```python
from build123d import *

# Parameters (mm, degrees)
SKETCH1_R                  = 1.79959
BASE_FLANGE1_DEPTH         = 2.3622
SKETCHED_START             = -88.9
SKETCHED_BEND1_OUTLINE_W   = 12.7
SKETCHED_BEND1_OUTLINE_H   = 2.3622
SKETCHED_BEND1_DEPTH       = 60.4012
SKETCHED_START_2           = -28.197410712
SKETCHED_BEND1_2_OUTLINE_W = 12.7
SKETCHED_BEND1_2_OUTLINE_H = 61.224283884
SKETCHED_BEND1_2_OUTLINE_R = 1.79959
SKETCHED_BEND1_2_DEPTH     = 2.060810712
SKETCHED_START_3           = -28.4988
SKETCHED_BEND1_3_OUTLINE_W = 12.7
SKETCHED_BEND1_3_OUTLINE_H = 61.224283884
SKETCHED_BEND1_3_OUTLINE_R = 1.79959
SKETCHED_BEND1_3_DEPTH     = 3.0988
SKETCHED_START_4           = 38.1
SKETCHED_BEND1_4_DEPTH     = 12.7
CUT_EXTRUDE1_REACH         = 88.233
SKETCH7_R                  = 1.55


with BuildPart() as part:
    # Base-Flange1: sheet metal written as solids
    # Sketch1 → Base-Flange1 (new body)
    with BuildSketch(Plane(origin=(0, 0, 0), x_dir=(1, 0, 0), z_dir=(0, 1, 0))):
        Polygon((50.8, 88.9), (50.8, 0), (0, 0), (0, 25.4), (38.1, 25.4), (38.1, 88.9), align=None)
        with Locations(Location((45.06468, 81.50352, 0), (0, 0, 270))):
            Circle(SKETCH1_R, mode=Mode.SUBTRACT)
        with Locations(Location((44.45, 35.56, 0), (0, 0, 270))):
            Circle(SKETCH1_R, mode=Mode.SUBTRACT)
    extrude(amount=-BASE_FLANGE1_DEPTH)

    # Sketched Bend1: read off the stored shape, not the designer's step
    # Sketched Bend1 outline → Sketched Bend1 (cut)
    with BuildSketch(Plane.XY.offset(SKETCHED_START)):
        with Locations((44.45, -1.1811)):
            Rectangle(SKETCHED_BEND1_OUTLINE_W, SKETCHED_BEND1_OUTLINE_H)
    extrude(amount=SKETCHED_BEND1_DEPTH, mode=Mode.SUBTRACT)

    # Sketched Bend1 2 outline → Sketched Bend1 2 (add)
    with BuildSketch(Plane.XY.offset(SKETCHED_START_2)):
        with Locations((44.45, -32.974341942)):
            Rectangle(SKETCHED_BEND1_2_OUTLINE_W, SKETCHED_BEND1_2_OUTLINE_H)
        with Locations((45.06468, -56.190003884)):
            Circle(SKETCHED_BEND1_2_OUTLINE_R, mode=Mode.SUBTRACT)
        with Locations((44.45, -10.246483884)):
            Circle(SKETCHED_BEND1_2_OUTLINE_R, mode=Mode.SUBTRACT)
    extrude(amount=SKETCHED_BEND1_2_DEPTH)

    # Sketched Bend1 3 outline → Sketched Bend1 3 (add)
    with BuildSketch(Plane.XY.offset(SKETCHED_START_3)):
        with Locations((44.45, -32.974341942)):
            Rectangle(SKETCHED_BEND1_3_OUTLINE_W, SKETCHED_BEND1_3_OUTLINE_H)
        with Locations((45.06468, -56.190003884)):
            Circle(SKETCHED_BEND1_3_OUTLINE_R, mode=Mode.SUBTRACT)
        with Locations((44.45, -10.246483884)):
            Circle(SKETCHED_BEND1_3_OUTLINE_R, mode=Mode.SUBTRACT)
    extrude(amount=SKETCHED_BEND1_3_DEPTH)

    # Sketched Bend1 4 outline → Sketched Bend1 4 (cut)
    with BuildSketch(Plane.YZ.offset(SKETCHED_START_4)):
        with BuildLine():
            ThreePointArc((0, -25.4), (-0.907617506, -27.591182494), (-3.0988, -28.4988))
            Line((-3.0988, -28.4988), (0, -28.4988))
            Line((0, -28.4988), (0, -25.4))
        make_face()
        with BuildLine():
            Line((-63.586483884, -26.1366), (-3.0988, -26.1366))
            ThreePointArc((-3.0988, -26.1366), (-2.577945145, -25.920854855), (-2.3622, -25.4))
            Line((-2.3622, -25.4), (-63.586483884, -25.4))
            Line((-63.586483884, -25.4), (-63.586483884, -26.1366))
        make_face()
    extrude(amount=SKETCHED_BEND1_4_DEPTH, mode=Mode.SUBTRACT)

    # Sketch7 → Cut-Extrude1 (cut, up to next)
    with BuildSketch(Plane(origin=(0, 0, 0), x_dir=(1, 0, 0), z_dir=(0, 1, 0)), mode=Mode.PRIVATE) as cut_extrude1_sk1:
        with Locations(Location((45.78, 20.828, 0), (0, 0, 270))):
            Circle(SKETCH7_R)
    cut_extrude1_tool1 = extrude(cut_extrude1_sk1.sketch, amount=-CUT_EXTRUDE1_REACH, mode=Mode.PRIVATE) & part.part
    # Sketch7 → Cut-Extrude1 (cut, up to next)
    with BuildSketch(Plane(origin=(0, 0, 0), x_dir=(1, 0, 0), z_dir=(0, 1, 0)), mode=Mode.PRIVATE) as cut_extrude1_sk2:
        with Locations(Location((5.08, 4.528, 0), (0, 0, 270))):
            Circle(SKETCH7_R)
    cut_extrude1_tool2 = extrude(cut_extrude1_sk2.sketch, amount=-CUT_EXTRUDE1_REACH, mode=Mode.PRIVATE) & part.part
    # Sketch7 → Cut-Extrude1 (cut, up to next)
    with BuildSketch(Plane(origin=(0, 0, 0), x_dir=(1, 0, 0), z_dir=(0, 1, 0)), mode=Mode.PRIVATE) as cut_extrude1_sk3:
        with Locations(Location((45.78, 4.528, 0), (0, 0, 270))):
            Circle(SKETCH7_R)
    cut_extrude1_tool3 = extrude(cut_extrude1_sk3.sketch, amount=-CUT_EXTRUDE1_REACH, mode=Mode.PRIVATE) & part.part
    # Sketch7 → Cut-Extrude1 (cut, up to next)
    with BuildSketch(Plane(origin=(0, 0, 0), x_dir=(1, 0, 0), z_dir=(0, 1, 0)), mode=Mode.PRIVATE) as cut_extrude1_sk4:
        with Locations(Location((5.08, 20.828, 0), (0, 0, 270))):
            Circle(SKETCH7_R)
    cut_extrude1_tool4 = extrude(cut_extrude1_sk4.sketch, amount=-CUT_EXTRUDE1_REACH, mode=Mode.PRIVATE) & part.part
    add(cut_extrude1_tool1.solids().sort_by_distance((45.78, 0, -20.828))[0], mode=Mode.SUBTRACT)
    add(cut_extrude1_tool2.solids().sort_by_distance((5.08, 0, -4.528))[0], mode=Mode.SUBTRACT)
    add(cut_extrude1_tool3.solids().sort_by_distance((45.78, 0, -4.528))[0], mode=Mode.SUBTRACT)
    add(cut_extrude1_tool4.solids().sort_by_distance((5.08, 0, -20.828))[0], mode=Mode.SUBTRACT)


solid = part.part
```
Verification items for the finished model (mm, model axes). A direction names the side the tool comes from. Coordinates: 2 decimals unless noted, no trailing zeros. Order: outer loops, then holes, each group sorted by start corner. A loop starts at its lowest first (then second) coordinate and runs counter-clockwise, first axis right, second up. Notation, with made-up numbers: (87, -6) - (146, -6) arc R29 ccw to (146, 32) - close; hole circle Ø11 at (2.25, -26). An arc over 180 degrees is marked (long way). Return JSON: item names as keys, results as strings.
(1) Go/stop test with flat-tipped pins: pin 1 (14 mm diameter, centred on x = 46, y = -41.5, fed in from +Z); pin 2 (2 mm diameter, centred on x = 45.06, y = -56.19, fed in from +Z); pin 3 (3.5 mm diameter, centred on x = 5.08, z = -20.828, fed in from -Y); pin 4 (1.9 mm diameter, centred on x = 12.5, y = -1.5, fed in from -Z). Record where each tip stops, or that it passes through.
Filled sheet:
{"pin 1": "stops at z = -26.14", "pin 2": "passes through", "pin 3": "stops at y = -2.36", "pin 4": "stops at z = -25.4"}
(2) Section check B-B, the plane z = -5.25. Record the cut outline in (x, y), and give its area (3 significant figures).
Filled sheet:
{"outline": "(0, -2.36) - (3.71, -2.36) - (3.71, 0) - (0, 0) - close; (6.45, -2.36) - (44.41, -2.36) - (44.41, 0) - (6.45, 0) - close; (47.15, -2.36) - (50.8, -2.36) - (50.8, 0) - (47.15, 0) - close", "area": "107 mm^2"}
(3) Section check D-D, the plane z = -18.25. Record the cut outline in (x, y).
Filled sheet:
{"outline": "(0, -2.36) - (50.8, -2.36) - (50.8, 0) - (0, 0) - close"}
(4) Access from +Z, -Z, +X, -X, +Y, -Y to the whole of each face (thin tool, end or side, straight path). Record for faces 4 (the flat face through (44, -34, -26.137)), 5 (the flat face through (0, -1, -13)), 6 (the flat face through (19, -1, -25.4)).
Filled sheet:
{"face 4": "+Z, +X, -X, -Y", "face 5": "+Z, -Z, -X, +Y, -Y", "face 6": "-Z, -X, +Y, -Y"}
(5) Thickness scan on line 1 along Y through (x, z) = (44.45, -27.5); line 2 along Y through (x, z) = (36.5, -3); line 3 along Z through (x, y) = (47.5, -45). Record the ranges inside material, lowest first.
Filled sheet:
{"line 1": "y = -63.59 to -57.88, -54.5 to -12.05, -8.45 to -0.82", "line 2": "y = -2.36 to 0", "line 3": "z = -28.5 to -26.14"}
(6) Section check A-A, the plane x = 5.08. Record the cut outline in (y, z), and give its area (3 significant figures).
Filled sheet:
{"outline": "(-2.36, -25.4) - (0, -25.4) - (0, -22.38) - (-2.36, -22.38) - close; (-2.36, -19.28) - (0, -19.28) - (0, -6.08) - (-2.36, -6.08) - close; (-2.36, -2.98) - (0, -2.98) - (0, 0) - (-2.36, 0) - close", "area": "45.4 mm^2"}
(7) Mould release check, pull along X, two halves, no side actions. Record for faces 1 (the flat face through (50.8, -23, -27)), 2 (the flat face through (44, -33, -28.499)), 3 (the cylindrical face through (47.317, -1.165, -21.03)): pulls with the +X half, pulls with the -X half, needs draft (parallel to the pull), parting line crosses it, or undercut.
Filled sheet:
{"face 1": "pulls with the +X half", "face 2": "needs draft", "face 3": "undercut"}
(8) Section check C-C, the plane y = -37. Record the cut outline in (x, z).
Filled sheet:
{"outline": "(38.1, -28.5) - (50.8, -28.5) - (50.8, -26.14) - (38.1, -26.14) - close"}
